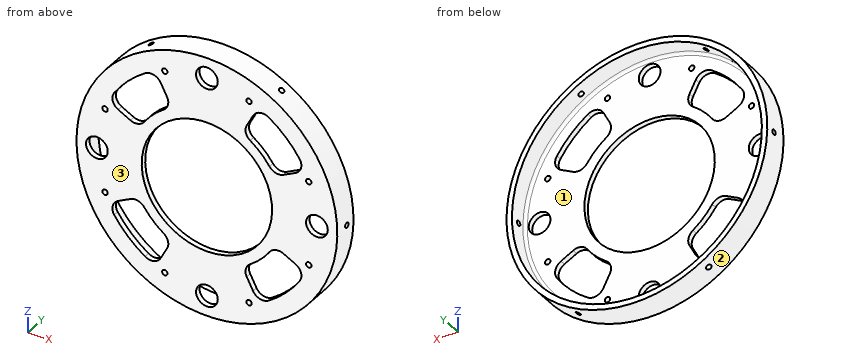
from build123d import *

# Parameters (mm, degrees)
SKETCH1_R           = 76.2
BOSS_EXTRUDE1_DEPTH = 16.256
SHELL1_T            = -3.175
FILLET1_R           = 1.5875
SKETCH2_R           = 38.1
CUT_EXTRUDE1_DEPTH  = 16.256
SKETCH3_R           = 1.524
CUT_EXTRUDE2_DEPTH  = 76.2
CIRPATTERN1_COUNT   = 6
CUT_EXTRUDE4_START  = -1.524
SKETCH5_R           = 76.2
CUT_EXTRUDE4_DEPTH  = 1.524
SKETCH6_R           = 6.35
CUT_EXTRUDE5_DEPTH  = 12.7
SKETCH7_R           = 1.5875
CUT_EXTRUDE6_DEPTH  = 6.35
SKETCH8_R           = 6.35
CUT_EXTRUDE7_DEPTH  = 6.35
CUT_EXTRUDE8_DEPTH  = 6.35
FILLET2_R           = 6.35


with BuildPart() as part:
    # Sketch1 → Boss-Extrude1 (new body)
    with BuildSketch(Plane(origin=(0, 0, 0), x_dir=(1, 0, 0), z_dir=(0, 1, 0))):
        with Locations(Location((0, 0, 0), (0, 0, 270))):
            Circle(SKETCH1_R)
    extrude(amount=BOSS_EXTRUDE1_DEPTH)

    # Shell1
    shell1_openings = [part.faces().sort_by_distance(p)[0] for p in [
        (0, 16.256, 0),
    ]]
    offset(amount=SHELL1_T, openings=shell1_openings, kind=Kind.INTERSECTION)

    # Fillet1
    fillet1_edges = [part.edges().sort_by_distance(p)[0] for p in [
        (0, 3.175, -73.025),
    ]]
    fillet(fillet1_edges, radius=FILLET1_R)

    # Sketch2 → Cut-Extrude1 (cut)
    with BuildSketch(Plane.XZ):
        with Locations(Location((0, 0, 0), (0, 0, 270))):
            Circle(SKETCH2_R)
    extrude(amount=-CUT_EXTRUDE1_DEPTH, mode=Mode.SUBTRACT)

    # Sketch3 → Cut-Extrude2 (cut)
    with BuildSketch(Plane(origin=(0, 0, 0), x_dir=(0, 0, -1), z_dir=(1, 0, 0))):
        with Locations((0, 8.636)):
            Circle(SKETCH3_R)
    cut_extrude2 = extrude(amount=-CUT_EXTRUDE2_DEPTH, mode=Mode.SUBTRACT)

    # CirPattern1: Cut-Extrude2 ×6 about axis
    cirpattern1_axis = Axis((0, 16.256, 0), (0, -1, 0))
    for i in range(1, CIRPATTERN1_COUNT):
        add(cut_extrude2.rotate(cirpattern1_axis, i * 360 / CIRPATTERN1_COUNT), mode=Mode.SUBTRACT)

    # Sketch5 → Cut-Extrude4 (cut)
    with BuildSketch(Plane(origin=(0, 16.256, 0), x_dir=(1, 0, 0), z_dir=(0, 1, 0)).offset(CUT_EXTRUDE4_START)):
        with Locations(Location((0, 0, 0), (0, 0, 270))):
            Circle(SKETCH5_R)
    extrude(amount=CUT_EXTRUDE4_DEPTH, mode=Mode.SUBTRACT)

    # Sketch6 → Cut-Extrude5 (cut)
    with BuildSketch(Plane(origin=(0, 3.175, 0), x_dir=(1, 0, 0), z_dir=(0, 1, 0))):
        with Locations(Location((0, 64.2874, 0), (0, 0, 270))):
            Circle(SKETCH6_R)
        with Locations(Location((0, -64.2874, 0), (0, 0, 270))):
            Circle(SKETCH6_R)
    extrude(amount=-CUT_EXTRUDE5_DEPTH, mode=Mode.SUBTRACT)

    # Sketch7 → Cut-Extrude6 (cut)
    with BuildSketch(Plane(origin=(0, 3.175, 0), x_dir=(1, 0, 0), z_dir=(0, 1, 0))):
        with Locations(Location((-24.6, 59.525, 0), (0, 0, 270))):
            Circle(SKETCH7_R)
        with Locations(Location((24.6, 59.525, 0), (0, 0, 270))):
            Circle(SKETCH7_R)
        with Locations(Location((24.6, -59.525, 0), (0, 0, 270))):
            Circle(SKETCH7_R)
        with Locations(Location((-24.6, -59.525, 0), (0, 0, 270))):
            Circle(SKETCH7_R)
        with Locations(Location((-59.525, -24.6, 0), (0, 0, 270))):
            Circle(SKETCH7_R)
        with Locations(Location((-59.525, 24.6, 0), (0, 0, 270))):
            Circle(SKETCH7_R)
        with Locations(Location((59.525, 24.6, 0), (0, 0, 270))):
            Circle(SKETCH7_R)
        with Locations(Location((59.525, -24.6, 0), (0, 0, 270))):
            Circle(SKETCH7_R)
    extrude(amount=-CUT_EXTRUDE6_DEPTH, mode=Mode.SUBTRACT)

    # Sketch8 → Cut-Extrude7 (cut)
    with BuildSketch(Plane(origin=(0, 3.175, 0), x_dir=(1, 0, 0), z_dir=(0, 1, 0))):
        with Locations(Location((0, 64.2874, 0), (0, 0, 270))):
            Circle(SKETCH8_R)
        with Locations(Location((0, -64.2874, 0), (0, 0, 270))):
            Circle(SKETCH8_R)
        with Locations(Location((64.2874, 0, 0), (0, 0, 270))):
            Circle(SKETCH8_R)
        with Locations(Location((-64.2874, 0, 0), (0, 0, 270))):
            Circle(SKETCH8_R)
    extrude(amount=-CUT_EXTRUDE7_DEPTH, mode=Mode.SUBTRACT)

    # Sketch9 → Cut-Extrude8 (cut)
    with BuildSketch(Plane(origin=(0, 3.175, 0), x_dir=(1, 0, 0), z_dir=(0, 1, 0))):
        with BuildLine():
            Line((-39.427631535, 20.524725858), (-57.733317604, 30.054062864))
            ThreePointArc((-57.733317604, 30.054062864), (-46.02381262, 46.02381262), (-30.054062864, 57.733317604))
            Line((-30.054062864, 57.733317604), (-20.524725858, 39.427631535))
            ThreePointArc((-20.524725858, 39.427631535), (-31.430896424, 31.430896424), (-39.427631535, 20.524725858))
        make_face()
        with BuildLine():
            Line((-20.524725858, -39.427631535), (-30.054062864, -57.733317604))
            ThreePointArc((-30.054062864, -57.733317604), (-46.02381262, -46.02381262), (-57.733317604, -30.054062864))
            Line((-57.733317604, -30.054062864), (-39.427631535, -20.524725858))
            ThreePointArc((-39.427631535, -20.524725858), (-31.430896424, -31.430896424), (-20.524725858, -39.427631535))
        make_face()
        with BuildLine():
            Line((39.427631535, -20.524725858), (57.733317604, -30.054062864))
            ThreePointArc((57.733317604, -30.054062864), (46.02381262, -46.02381262), (30.054062864, -57.733317604))
            Line((30.054062864, -57.733317604), (20.524725858, -39.427631535))
            ThreePointArc((20.524725858, -39.427631535), (31.430896424, -31.430896424), (39.427631535, -20.524725858))
        make_face()
        with BuildLine():
            Line((20.524725858, 39.427631535), (30.054062864, 57.733317604))
            ThreePointArc((30.054062864, 57.733317604), (46.02381262, 46.02381262), (57.733317604, 30.054062864))
            Line((57.733317604, 30.054062864), (39.427631535, 20.524725858))
            ThreePointArc((39.427631535, 20.524725858), (31.430896424, 31.430896424), (20.524725858, 39.427631535))
        make_face()
    extrude(amount=-CUT_EXTRUDE8_DEPTH, mode=Mode.SUBTRACT)

    # Fillet2
    fillet2_edges = [part.edges().sort_by_distance(p)[0] for p in [
        (-30.054062864, 1.5875, 57.733317604),
        (-57.733317604, 1.5875, 30.054062864),
        (-39.427631535, 1.5875, 20.524725858),
        (-20.524725858, 1.5875, 39.427631535),
        (-57.733317604, 1.5875, -30.054062864),
        (-30.054062864, 1.5875, -57.733317604),
        (-20.524725858, 1.5875, -39.427631535),
        (-39.427631535, 1.5875, -20.524725858),
        (20.524725858, 1.5875, 39.427631535),
        (39.427631535, 1.5875, 20.524725858),
        (57.733317604, 1.5875, 30.054062864),
        (30.054062864, 1.5875, 57.733317604),
        (30.054062864, 1.5875, -57.733317604),
        (57.733317604, 1.5875, -30.054062864),
        (39.427631535, 1.5875, -20.524725858),
        (20.524725858, 1.5875, -39.427631535),
    ]]
    fillet(fillet2_edges, radius=FILLET2_R)


solid = part.part
Can you work these out from the model? Positions are in its coordinate system, mm. Face numbers are marked on the shaded views. Give positions to 0.01 mm unless a question says otherwise; leave off trailing zeros. Loops run counter-clockwise (first coordinate to the right, second up) from the corner with the lowest first, then second, coordinate; pieces in that order, holes last. Notation, with made-up numbers: (60.25, -8.75) -> (94.25, -8.75) arc R14 ccw to (94.25, 18.25) -> close; hole circle Ø4 at (-36, -19). An arc over 180 degrees is marked (long way). Return JSON: item names as keys, results as strings.
Q1. For pin 1 Ø2 at (y, z) = (2.5, -37.5) entering from -X; pin 2 Ø1.8 at (y, z) = (8.636, 0) entering from +X; pin 3 Ø3 at (y, z) = (11, -27.5) entering from -X; pin 4 Ø1 at (x, y) = (-40, 8) entering from +Z, each with a flat end and sliding along its axis, tell me the tip position at first contact or that it passes through.
Checks:
{"pin 1": "stops at x = -66.89", "pin 2": "passes through", "pin 3": "stops at x = -71.63", "pin 4": "stops at z = 65.16"}
Q2. I want a section at B-B, the plane y = 12.5. List the corners of the cut face in (x, z) for me (3 decimals).
Checks:
{"outline": "circle Ø152.4 at (0, 0); hole circle Ø146.05 at (0, 0)"}
Q3. We'd pull the mould along X, two halves only. Please class the marked faces 1, 2 and 3: released by +X, released by -X, zero draft, split by the parting line, or undercut.
Checks:
{"face 1": "undercut", "face 2": "split by the parting line", "face 3": "zero draft"}
Q4. I want a section at C-C, the plane z = 30. Count the separate pieces of the cut face and the enclosed holes in it, then the cut area to 3 significant figures.
Checks:
{"separate pieces": "4", "enclosed holes": "0", "area": "238 mm2"}
Q5. I need wall thicknesses on probe 1 along X at (y, z) = (2, 0); probe 2 along X at (y, z) = (10.75, 0) (3 decimals); probe 3 along X at (y, z) = (2.75, 53.5). Which ranges of each line are inside material? Lowest first, please.
Checks:
{"probe 1": "x = -76.2 to -70.64, -57.94 to -38.1, 38.1 to 57.94, 70.64 to 76.2", "probe 2": "x = -76.2 to -73.025, 73.025 to 76.2", "probe 3": "x = -54.26 to -37.07, -28.26 to 28.26, 37.07 to 54.26"}
Q6. I want a section at A-A, the plane x = 0. List the corners of the cut face in (y, z) for me (1 decimal), then the cut area to 3 significant figures.
Checks:
{"outline": "(0, -76.2) -> (14.7, -76.2) -> (14.7, -73) -> (4.8, -73) arc R1.6 cw to (3.2, -71.4) -> (3.2, -70.6) -> (0, -70.6) -> close; (0, -57.9) -> (3.2, -57.9) -> (3.2, -38.1) -> (0, -38.1) -> close; (0, 38.1) -> (3.2, 38.1) -> (3.2, 57.9) -> (0, 57.9) -> close; (0, 70.6) -> (3.2, 70.6) -> (3.2, 71.4) arc R1.6 cw to (4.8, 73) -> (14.7, 73) -> (14.7, 76.2) -> (0, 76.2) -> close", "area": "236 mm2"}
